```python
from build123d import *

# Parameters (mm, degrees)
F2_DEPTH = 17
F3_T     = -2
F1_R     = 1.55
F4_DEPTH = 2
F5_DEPTH = 25
F6_D     = 3
F7_R     = 1.99999


# Not quite as in the source:
# - a fillet or chamfer is up to 0.001 mm smaller than in the source, because OpenCascade refuses the exact size


with BuildPart() as f2:
    # F1 (on Top) → F2 (new body)
    with BuildSketch(Plane.XY):
        with BuildLine():
            ThreePointArc((73.2924652381, 31.6927541938), (72.4137855817, 33.8140745374), (70.2924652381, 34.6927541938))
            Line((70.2924652381, 34.6927541938), (-70.2924652381, 34.6927541938))
            ThreePointArc((-70.2924652381, 34.6927541938), (-72.4137855817, 33.8140745374), (-73.2924652381, 31.6927541938))
            Line((-73.2924652381, 31.6927541938), (-73.2924652381, -31.6927541938))
            ThreePointArc((-73.2924652381, -31.6927541938), (-72.4137855817, -33.8140745374), (-70.2924652381, -34.6927541938))
            Line((-70.2924652381, -34.6927541938), (70.2924652381, -34.6927541938))
            ThreePointArc((70.2924652381, -34.6927541938), (72.4137855817, -33.8140745374), (73.2924652381, -31.6927541938))
            Line((73.2924652381, -31.6927541938), (73.2924652381, 31.6927541938))
        make_face()
        with BuildLine():
            ThreePointArc((65.2924652381, -23.6927541938), (64.4137855817, -25.8140745374), (62.2924652381, -26.6927541938))
            Line((62.2924652381, -26.6927541938), (-62.2924652381, -26.6927541938))
            ThreePointArc((-62.2924652381, -26.6927541938), (-64.4137855817, -25.8140745374), (-65.2924652381, -23.6927541938))
            Line((-65.2924652381, -23.6927541938), (-65.2924652381, 23.6927541938))
            ThreePointArc((-65.2924652381, 23.6927541938), (-64.4137855817, 25.8140745374), (-62.2924652381, 26.6927541938))
            Line((-62.2924652381, 26.6927541938), (62.2924652381, 26.6927541938))
            ThreePointArc((62.2924652381, 26.6927541938), (64.4137855817, 25.8140745374), (65.2924652381, 23.6927541938))
            Line((65.2924652381, 23.6927541938), (65.2924652381, -23.6927541938))
        make_face(mode=Mode.SUBTRACT)
        with BuildLine():
            Line((-62.2924652381, -26.6927541938), (62.2924652381, -26.6927541938))
            ThreePointArc((62.2924652381, -26.6927541938), (64.4137855817, -25.8140745374), (65.2924652381, -23.6927541938))
            Line((65.2924652381, -23.6927541938), (65.2924652381, 23.6927541938))
            ThreePointArc((65.2924652381, 23.6927541938), (64.4137855817, 25.8140745374), (62.2924652381, 26.6927541938))
            Line((62.2924652381, 26.6927541938), (-62.2924652381, 26.6927541938))
            ThreePointArc((-62.2924652381, 26.6927541938), (-64.4137855817, 25.8140745374), (-65.2924652381, 23.6927541938))
            Line((-65.2924652381, 23.6927541938), (-65.2924652381, -23.6927541938))
            ThreePointArc((-65.2924652381, -23.6927541938), (-64.4137855817, -25.8140745374), (-62.2924652381, -26.6927541938))
        make_face()
    extrude(amount=-F2_DEPTH)

    # F3
    f3_openings = [f2.faces().sort_by_distance(p)[0] for p in [
        (0, 0, -17),
    ]]
    offset(amount=F3_T, openings=f3_openings)

    # F1 (on Top) → F4 (join)
    with BuildSketch(Plane.XY):
        with BuildLine():
            Line((-70.2924652381, 34.6927541938), (70.2924652381, 34.6927541938))
            ThreePointArc((70.2924652381, 34.6927541938), (72.4137855817, 33.8140745374), (73.2924652381, 31.6927541938))
            Line((73.2924652381, 31.6927541938), (73.2924652381, 34.6927541938))
            Line((73.2924652381, 34.6927541938), (73.2924652381, 46.6927541938))
            ThreePointArc((73.2924652381, 46.6927541938), (72.4137855817, 48.8140745374), (70.2924652381, 49.6927541938))
            Line((70.2924652381, 49.6927541938), (-70.2924652381, 49.6927541938))
            ThreePointArc((-70.2924652381, 49.6927541938), (-72.4137855817, 48.8140745374), (-73.2924652381, 46.6927541938))
            Line((-73.2924652381, 46.6927541938), (-73.2924652381, 34.6927541938))
            Line((-73.2924652381, 34.6927541938), (-73.2924652381, 31.6927541938))
            ThreePointArc((-73.2924652381, 31.6927541938), (-72.4137855817, 33.8140745374), (-70.2924652381, 34.6927541938))
        make_face()
        with Locations((-66.2924652381, 42.1927541938)):
            Circle(F1_R, mode=Mode.SUBTRACT)
        with Locations((0, 42.1927541938)):
            Circle(F1_R, mode=Mode.SUBTRACT)
        with Locations((66.2924652381, 42.1927541938)):
            Circle(F1_R, mode=Mode.SUBTRACT)
    extrude(amount=-F4_DEPTH)

    # F1 (on Top) → F5 (cut)
    with BuildSketch(Plane.XY):
        with BuildLine():
            Line((-62.2924652381, -26.6927541938), (62.2924652381, -26.6927541938))
            ThreePointArc((62.2924652381, -26.6927541938), (64.4137855817, -25.8140745374), (65.2924652381, -23.6927541938))
            Line((65.2924652381, -23.6927541938), (65.2924652381, 23.6927541938))
            ThreePointArc((65.2924652381, 23.6927541938), (64.4137855817, 25.8140745374), (62.2924652381, 26.6927541938))
            Line((62.2924652381, 26.6927541938), (-62.2924652381, 26.6927541938))
            ThreePointArc((-62.2924652381, 26.6927541938), (-64.4137855817, 25.8140745374), (-65.2924652381, 23.6927541938))
            Line((-65.2924652381, 23.6927541938), (-65.2924652381, -23.6927541938))
            ThreePointArc((-65.2924652381, -23.6927541938), (-64.4137855817, -25.8140745374), (-62.2924652381, -26.6927541938))
        make_face()
    extrude(amount=-F5_DEPTH, mode=Mode.SUBTRACT)

    # F6 (through all)
    with Locations(Plane.XY):
        with Locations((-66.2924652381, 27.6927541938), (66.2980739571, 27.6781461437), (66.291973394, -27.6938535203), (-66.2985658012, -27.6792454701)):
            Hole(F6_D / 2)

    # F7 (radius 2 in the source; OpenCascade refuses exactly that, so slightly less here)
    f7_edges = [f2.edges().sort_by_distance(p)[0] for p in [
        (-73.292465, 7.5, 0),
    ]]
    fillet(f7_edges, radius=F7_R)


solid = f2.part
```
Can you work these out from the model? Positions are in its coordinate system, mm. A direction names the side the tool comes from. Coordinates: 2 decimals unless noted, no trailing zeros. Loops run counter-clockwise (first coordinate to the right, second up) from the corner with the lowest first, then second, coordinate; pieces in that order, holes last.
Item 1: Suppose I cut it at D-D (x = 0). State how many separate pieces and enclosed holes the cut face has, then the cut area to 3 significant figures.
Answers below:
separate pieces: 3
enclosed holes: 0
area: 114 mm2
Item 2: If we mould it in two halves opening along X, with no side actions, what happens to faces 1 (the face through (5, 32, 0)), 2 (the face through (67.49, 26.77, -1.01)), 3 (the face through (73.292, -2, -9))? For each: released by +X, released by -X, zero draft, split by the parting line, or undercut.
Answers below:
face 1: zero draft
face 2: undercut
face 3: released by +X
Item 3: Please list where these lines run through material, in increasing order: L1, parallel to Y at x = -24, z = -8.25; L2, parallel to X at y = 20, z = -14.5; L3, parallel to Y at x = 0, z = -0.35.
Answers below:
L1: y = -34.69 to -32.69, 32.69 to 34.69
L2: x = -73.29 to -71.29, 71.29 to 73.29
L3: y = -33.82 to -26.69, 26.69 to 40.64, 43.74 to 48.82
Item 4: Suppose I cut it at B-B (y = 2.5). Please give me the cut outline in (x, z).
Answers below:
outline: (-73.29, -17) - (-71.29, -17) - (-71.29, -2) - (-65.29, -2) - (-65.29, 0) - (-71.29, 0) arc R2 ccw to (-73.29, -2) - close; (65.29, -2) - (71.29, -2) - (71.29, -17) - (73.29, -17) - (73.29, -2) arc R2 ccw to (71.29, 0) - (65.29, 0) - close
Item 5: I'm going to push flat-ended pins straight in: pin 1 (2.5 mm diameter, centred on x = 66.3, y = 27.68, fed in from +Z); pin 2 (4 mm diameter, centred on x = -66.29, y = 27.69, fed in from -Z); pin 3 (0.6 mm diameter, centred on y = 4, z = -0.5, fed in from -X); pin 4 (0.6 mm diameter, centred on x = 3.5, z = -1, fed in from -Y). Where does each tip first touch, or does it pass through?
Answers below:
pin 1: passes through
pin 2: stops at z = -2
pin 3: stops at x = -72.89
pin 4: stops at y = -34.57
Item 6: Which directions (+Z, -Z, +X, -X, +Y, -Y) give clear straight access to the entire face, cutting with the end or side of a thin tool? Please do faces 4 (the face through (0, 27, -2)), 5 (the face through (64.44, 25.79, -0.99)), 6 (the face through (1, 34.693, -9)).
Answers below:
face 4: -Z
face 5: +Z, -Z
face 6: -Z, +X, -X, +Y
Item 7: Suppose I cut it at A-A (z = -7). Please give me the cut outline in (x, y).
Answers below:
outline: (-73.29, -31.69) arc R3 ccw to (-70.29, -34.69) - (70.29, -34.69) arc R3 ccw to (73.29, -31.69) - (73.29, 31.69) arc R3 ccw to (70.29, 34.69) - (-70.29, 34.69) arc R3 ccw to (-73.29, 31.69) - close; hole (-71.29, -31.69) arc R1 ccw to (-70.29, -32.69) - (70.29, -32.69) arc R1 ccw to (71.29, -31.69) - (71.29, 31.69) arc R1 ccw to (70.29, 32.69) - (-70.29, 32.69) arc R1 ccw to (-71.29, 31.69) - close
